Verification items for this drawing (mm, ordinates from the low corner). Give positions to 0.01 mm unless a question says otherwise; leave off trailing zeros. Order: outer loops, then holes, each group sorted by start corner. A loop starts at its lowest first (then second) coordinate and runs counter-clockwise, first axis right, second up.
(1) Sectioned sample at A-A on z = 38.1. Record the cut outline in (x, y) (1 decimal).
(2) Gauge pin test, flat ends, axial feed: pin 1 (4 mm diameter, centred on x = 38.1, z = 38.1, fed in from -Y); pin 2 (1 mm diameter, centred on x = 36, y = 2, fed in from -Z). Record the tip position at first contact, or that the pin passes through.
(3) Scan lines: L1, parallel to X at y = 0.9, z = 38.1; L2, parallel to X at y = 2.4, z = 12.7; L3, parallel to Z at x = 38.1, y = 2. Record each from-to range of solid material in increasing order.
(4) Sectioned sample at D-D on x = 63.5. Record the cut outline in (y, z) (1 decimal), plus the area to 3 significant figures.
(5) Sectioned sample at B-B on y = 2.3. Record the cut outline in (x, z).
(6) Sectioned sample at C-C on z = 12.7. Record the cut outline in (x, y) (1 decimal).
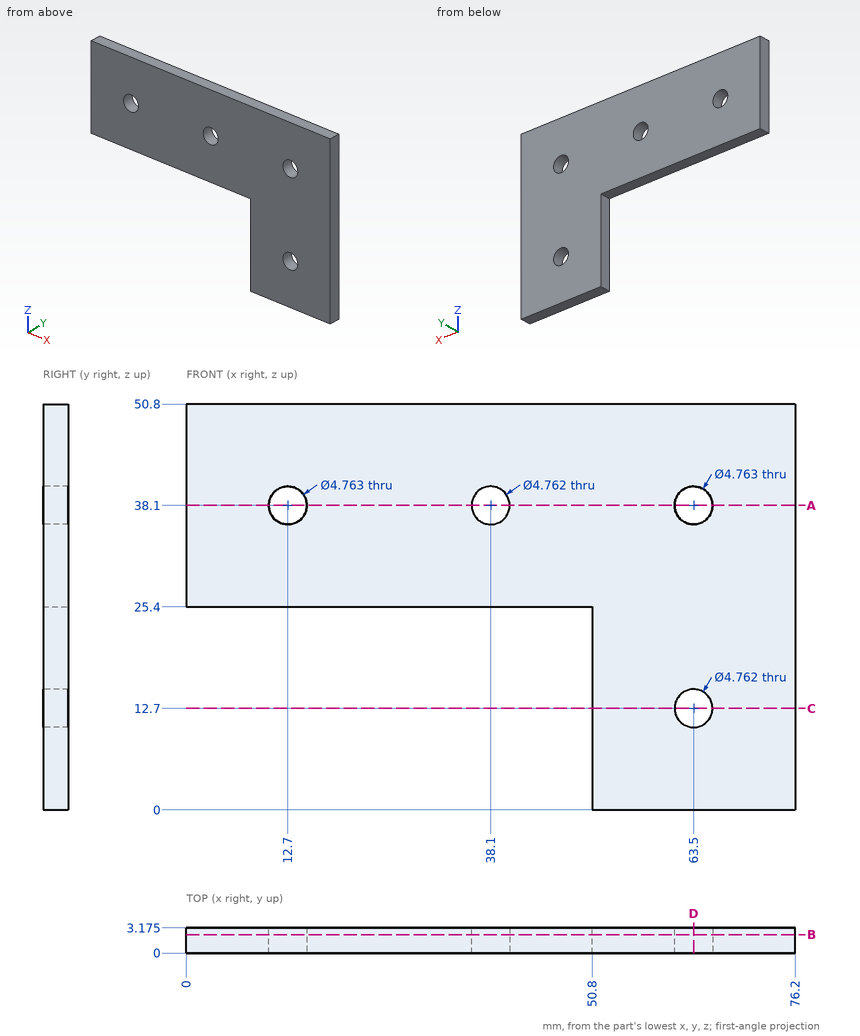
Ans:
1. outline: (0, 0) - (10.3, 0) - (10.3, 3.2) - (0, 3.2) - close; (15.1, 0) - (35.7, 0) - (35.7, 3.2) - (15.1, 3.2) - close; (40.5, 0) - (61.1, 0) - (61.1, 3.2) - (40.5, 3.2) - close; (65.9, 0) - (76.2, 0) - (76.2, 3.2) - (65.9, 3.2) - close
2. pin 1: passes through
2. pin 2: stops at z = 25.4
3. L1: x = 0 to 10.32, 15.08 to 35.72, 40.48 to 61.12, 65.88 to 76.2
3. L2: x = 50.8 to 61.12, 65.88 to 76.2
3. L3: z = 25.4 to 35.72, 40.48 to 50.8
4. outline: (0, 0) - (3.2, 0) - (3.2, 10.3) - (0, 10.3) - close; (0, 15.1) - (3.2, 15.1) - (3.2, 35.7) - (0, 35.7) - close; (0, 40.5) - (3.2, 40.5) - (3.2, 50.8) - (0, 50.8) - close
4. area: 131 mm2
5. outline: (0, 25.4) - (50.8, 25.4) - (50.8, 0) - (76.2, 0) - (76.2, 50.8) - (0, 50.8) - close; hole circle Ø4.76 at (12.7, 38.1); hole circle Ø4.76 at (38.1, 38.1); hole circle Ø4.76 at (63.5, 12.7); hole circle Ø4.76 at (63.5, 38.1)
6. outline: (50.8, 0) - (61.1, 0) - (61.1, 3.2) - (50.8, 3.2) - close; (65.9, 0) - (76.2, 0) - (76.2, 3.2) - (65.9, 3.2) - close
